from build123d import *

# Parameters (mm, degrees)
SKETCH3_W                = 25.4
SKETCH3_H                = 25.4
SKETCH3_W_2              = 22.225
SKETCH3_H_2              = 22.225
BOSS_EXTRUDE1_DEPTH      = 76.2
BOSS_EXTRUDE1_DEPTH_BACK = 76.2


with BuildPart() as part:
    # Sketch3 → Boss-Extrude1 (new body, two sides)
    with BuildSketch(Plane.XY) as boss_extrude1_sk:
        Rectangle(SKETCH3_W, SKETCH3_H)
        Rectangle(SKETCH3_W_2, SKETCH3_H_2, mode=Mode.SUBTRACT)
    extrude(amount=BOSS_EXTRUDE1_DEPTH)
    extrude(boss_extrude1_sk.sketch, amount=-BOSS_EXTRUDE1_DEPTH_BACK)


solid = part.part
Work out the finished part from the listing and answer in its coordinate system (mm). A direction names the side the tool comes from. Round coordinates to 2 decimals unless told otherwise and drop trailing zeros. Write each loop counter-clockwise with the first axis right and the second up, starting at its lowest first coordinate (ties: lowest second). Pieces come first, ordered by that corner, then holes.
1) A tool of negligible diameter and unlimited length cuts with its end or side. For faces 1 (the flat face through (-11.3, 0.1, -76.2)), 2 (the flat face through (0, -11.112, 1)), from which of +Z, -Z, +X, -X, +Y, -Y can it reach the whole face along a straight path? Write none if from no direction.
2) A cutting plane is placed at A-A (x = -1). Give the vertices of the cut face in (y, z).
3) The mould has two halves that part along X. Classify faces 3 (the flat face through (-12.7, 0, 1)), 4 (the flat face through (12.7, 0, 1)), 5 (the flat face through (11.112, 0, 1)): pulls with the +X half, pulls with the -X half, needs draft (parallel to the pull), parting line crosses it, or undercut.
4) A straight line is drawn through the part: line 1 (X direction, y = 1.5, z = -50.5). Find the intervals that lie inside material, in ascending order.
5) Given pin 1 Ø10 at (x, y) = (4.5, 9) entering from +Z; pin 2 Ø8 at (x, y) = (-3, -3.5) entering from -Z, each flat-ended and moving along its own axis, determine where each tip first touches the part or whether it passes through.
6) A cutting plane is placed at B-B (z = -3.5). Give the vertices of the cut face in (x, y), plus the area to 3 significant figures.
Completed:
1. face 1: -Z, +X, -X, +Y, -Y
1. face 2: +Z, -Z
2. outline: (-12.7, -76.2) - (-11.11, -76.2) - (-11.11, 76.2) - (-12.7, 76.2) - close; (11.11, -76.2) - (12.7, -76.2) - (12.7, 76.2) - (11.11, 76.2) - close
3. face 3: pulls with the -X half
3. face 4: pulls with the +X half
3. face 5: undercut
4. line 1: x = -12.7 to -11.11, 11.11 to 12.7
5. pin 1: stops at z = 76.2
5. pin 2: passes through
6. outline: (-12.7, -12.7) - (12.7, -12.7) - (12.7, 12.7) - (-12.7, 12.7) - close; hole (-11.11, -11.11) - (11.11, -11.11) - (11.11, 11.11) - (-11.11, 11.11) - close
6. area: 151 mm2
